Answer from the drawing. Dimensions are ordinates in mm from the lowest x, y and z of the part. Coordinates: 2 decimals unless noted, no trailing zeros. Write each loop counter-clockwise with the first axis right and the second up, starting at its lowest first coordinate (ties: lowest second). Pieces come first, ordered by that corner, then holes.
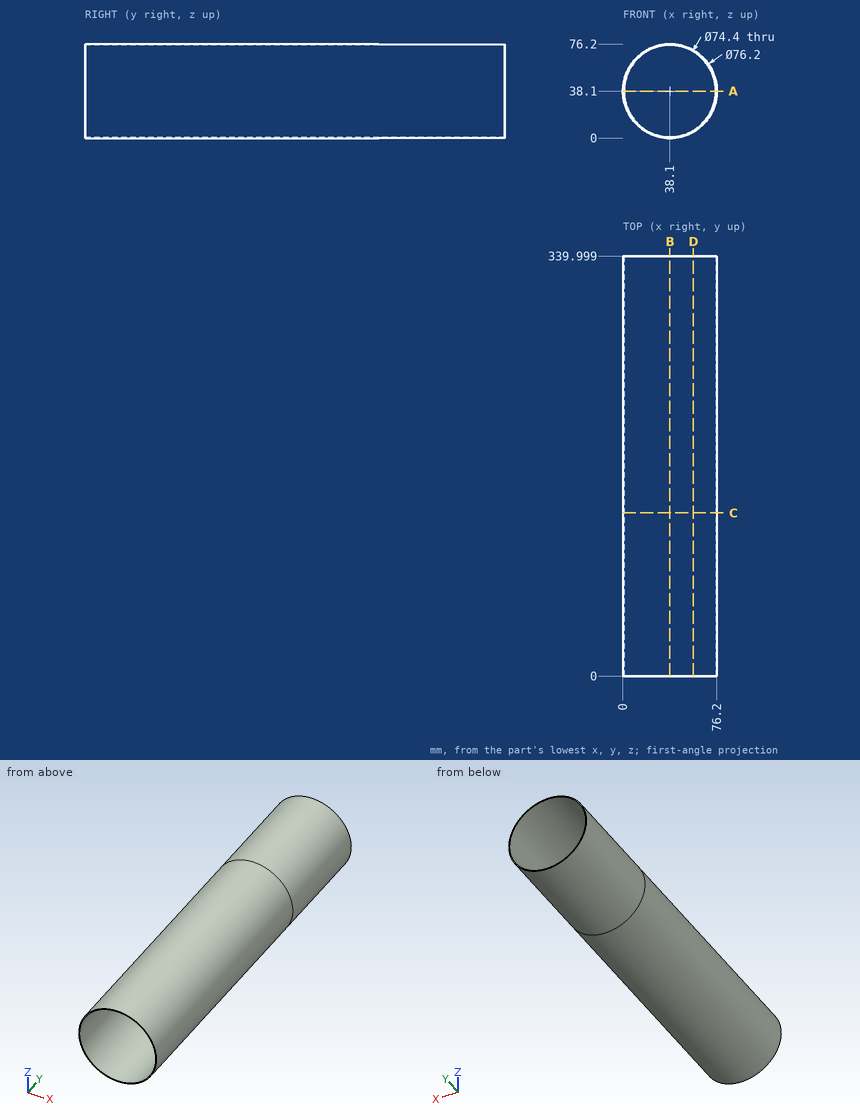
(1) Section A-A, the plane z = 38.1 is taken. Write down the section's boundary in (x, y), plus the area to 3 significant figures.
(2) Each of these flat-tipped pins is pushed along its axis until it touches: pin 1 (4 mm diameter, centred on x = 16, y = 294.5, fed in from +Z); pin 2 (1 mm diameter, centred on x = 59.5, y = 73.5, fed in from -Z); pin 3 (10 mm diameter, centred on y = 137, z = 53, fed in from -X). Where does it stop, or does it pass through?
(3) Section D-D, the plane x = 57 is taken. Write down the section's boundary in (y, z).
(4) Section C-C, the plane y = 132 is taken. Write down the section's boundary in (x, z), plus the area to 3 significant figures.
(5) Find the intervals of material crossed by probe 1 along Z at (x, y) = (38, 204); probe 2 along X at (y, z) = (169, 18), in increasing order.
(6) Section B-B, the plane x = 38.1 is taken. Write down the section's boundary in (y, z).
Solution:
1. outline: (0, 0) - (0.9, 0) - (0.9, 340) - (0, 340) - close; (75.3, 0) - (76.2, 0) - (76.2, 340) - (75.3, 340) - close
1. area: 612 mm2
2. pin 1: stops at z = 70.47
2. pin 2: stops at z = 6.24
2. pin 3: stops at x = 1.31
3. outline: (0, 5.02) - (340, 5.02) - (340, 6.06) - (0, 6.06) - close; (0, 70.14) - (340, 70.14) - (340, 71.18) - (0, 71.18) - close
4. outline: circle Ø76.2 at (38.1, 38.1); hole circle Ø74.4 at (38.1, 38.1)
4. area: 213 mm2
5. probe 1: z = 0 to 0.9, 75.3 to 76.2
5. probe 2: x = 5.73 to 6.8, 69.4 to 70.47
6. outline: (0, 0) - (340, 0) - (340, 0.9) - (0, 0.9) - close; (0, 75.3) - (340, 75.3) - (340, 76.2) - (0, 76.2) - close
